Study the drawing (mm; zero at the part's minimum x, y, z) and answer. A direction names the side the tool comes from. Round coordinates to 2 decimals unless told otherwise and drop trailing zeros. Order: outer loops, then holes, each group sorted by start corner. A loop starts at its lowest first (then second) coordinate and runs counter-clockwise, first axis right, second up. Notation, with made-up numbers: (-13.75, 55) - (19.25, 55) arc R12 ccw to (19.25, 77) - close; hole circle Ø10 at (-12.75, 42.25). An arc over 180 degrees is marked (long way). Put each result on its own line as item: value. Start each with the question number.
Q1. Each of these flat-tipped pins is pushed along its axis until it touches: pin 1 Ø0.6 at (x, z) = (0.5, 2.5) entering from +Y; pin 2 Ø7 at (y, z) = (23, 2.5) entering from -X; pin 3 Ø8 at (x, y) = (39, 38) entering from -Z (3 decimals). Where does it stop, or does it pass through?
Q2. Section D-D on z = 5.5 is taken. Give the vertices of the cut face in (x, y), then the cut area to 3 significant figures.
Q3. Section B-B on y = 25.5 is taken. Give the vertices of the cut face in (x, z) (3 decimals).
Q4. For a pull along X with two mould halves and no side action, classify the marked faces 1, 2 and 3 as pulls with the +X half, pulls with the -X half, needs draft (parallel to the pull), parting line crosses it, or undercut.
Q5. Find the intervals of material crossed by line 1 along X through (y, z) = (39, 10); line 2 along Y through (x, z) = (12.9, 11.25); line 3 along Y through (x, z) = (15, 3), in increasing order. Write a range as from..to.
Q6. Which of the six approach directions +Z, -Z, +X, -X, +Y, -Y give full straight-line access (tool end or side, diameter ignored) to the marked faces 4 and 5?
Q7. Section A-A on x = 8.5 is taken. Give the vertices of the cut face in (y, z) (3 decimals), then the cut area to 3 significant figures.
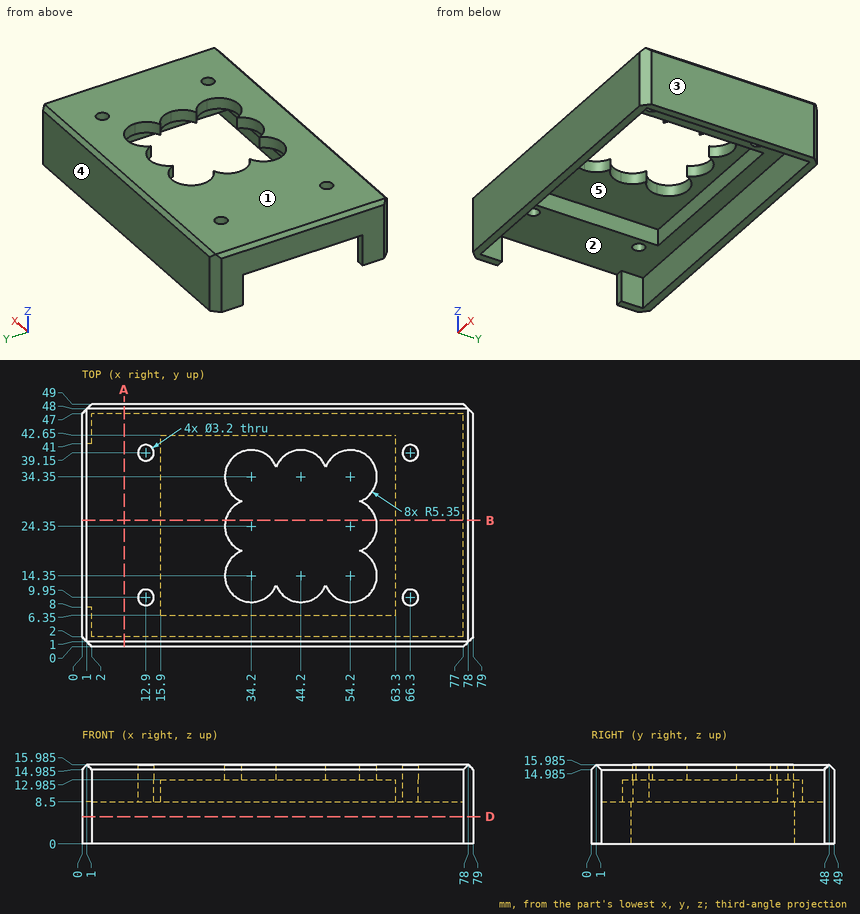
Findings:
1. pin 1: y = 47.8
1. pin 2: x = 77
1. pin 3: z = 12.985
2. outline: (0, 2) - (2, 0) - (77, 0) - (79, 2) - (79, 47) - (77, 49) - (2, 49) - (0, 47) - (0, 41) - (2, 41) - (2, 47) - (77, 47) - (77, 2) - (2, 2) - (2, 8) - (0, 8) - close
2. area: 422 mm2
3. outline: (0, 8.5) - (15.9, 8.5) - (15.9, 12.985) - (28.975, 12.985) - (28.975, 15.985) - (1, 15.985) - (0, 14.985) - close; (59.425, 12.985) - (63.3, 12.985) - (63.3, 8.5) - (77, 8.5) - (77, 0) - (79, 0) - (79, 14.985) - (78, 15.985) - (59.425, 15.985) - close
4. face 1: needs draft
4. face 2: undercut
4. face 3: pulls with the +X half
5. line 1: 0..11.31, 14.49..15.9, 63.3..64.71, 67.89..79
5. line 2: 0..8.35, 11.55..37.55, 40.75..49
5. line 3: 0..2, 47..49
6. face 4: +Z, -Z, +X, -X, +Y
6. face 5: -Z
7. outline: (0, 0) - (2, 0) - (2, 8.5) - (47, 8.5) - (47, 0) - (49, 0) - (49, 14.985) - (48, 15.985) - (1, 15.985) - (0, 14.985) - close
7. area: 400 mm2
